Work out the finished part from the listing and answer in its coordinate system (mm). A direction names the side the tool comes from. Coordinates: 2 decimals unless noted, no trailing zeros. Order: outer loops, then holes, each group sorted by start corner. A loop starts at its lowest first (then second) coordinate and runs counter-clockwise, first axis right, second up. Notation, with made-up numbers: (66, -9) -> (101, -9) arc R26 ccw to (101, 5) -> close; hole circle Ø4 at (31.5, -3.75). An arc over 180 degrees is marked (long way). Use one line per item in the form item = value.
from build123d import *

# Parameters (mm, degrees)
BOSS_EXTRUDE1_DEPTH = 900
BOSS_EXTRUDE7_DEPTH = 154.432
BOSS_EXTRUDE9_DEPTH = 86.012287
FILLET1_R           = 2.54
FILLET2_R           = 2.54


with BuildPart() as part:
    # Sketch1 → Boss-Extrude1 (new body)
    with BuildSketch(Plane.XY):
        Polygon((0, -0.000240533), (154.432, -0.000240533), (154.432, -11.557240533), (81.28, -11.557240533), (81.28, -150.495240533), (154.432, -150.495240533), (154.432, -162.052240533), (0, -162.052240533), (0, -150.495240533), (73.152, -150.495240533), (73.152, -11.557240533), (0, -11.557240533), align=None)
    extrude(amount=BOSS_EXTRUDE1_DEPTH)

    # Sketch4 → Boss-Extrude7 (add)
    with BuildSketch(Plane(origin=(154.432, 0, 0), x_dir=(0, 0, -1), z_dir=(1, 0, 0))):
        Polygon((-900, -0.000240533), (-914.177712902, -162.052240533), (-900, -162.052240533), align=None)
    extrude(amount=-BOSS_EXTRUDE7_DEPTH)

    # Sketch6 → Boss-Extrude9 (add)
    with BuildSketch(Plane(origin=(0, 0, 0), x_dir=(-1, 0, 0), z_dir=(0, 0, -1))):
        Polygon((0, -11.557240533), (0, -0.000240533), (-154.432, -0.000240533), (-154.432, -11.557240533), (-81.28, -11.557240533), (-81.28, -150.495240533), (-154.432, -150.495240533), (-154.432, -162.052240533), (0, -162.052240533), (0, -150.495240533), (-73.152, -150.495240533), (-73.152, -11.557240533), align=None)
    extrude(amount=BOSS_EXTRUDE9_DEPTH)

    # Fillet1
    fillet1_edges = [part.edges().sort_by_distance(p)[0] for p in [
        (36.576, -150.495240533, 900),
        (117.856, -150.495240533, 900),
        (117.856, -11.557240533, 900),
        (77.216, -162.052240533, 914.177712902),
        (77.216, -0.000240533, 900),
        (36.576, -11.557240533, 900),
    ]]
    fillet(fillet1_edges, radius=FILLET1_R)

    # Fillet2
    fillet2_edges = [part.edges().sort_by_distance(p)[0] for p in [
        (77.216, -162.052240533, -86.012287),
    ]]
    fillet(fillet2_edges, radius=FILLET2_R)


solid = part.part
(1) Which of the six approach directions +Z, -Z, +X, -X, +Y, -Y give full straight-line access (tool end or side, diameter ignored) to faces 1 (the flat face through (81.28, -80, 414)), 2 (the flat face through (78, -56, -86.012)), 3 (the flat face through (37, -82, 900))?
Data:
face_1 = -Z, +X
face_2 = -Z, +X, -X, +Y, -Y
face_3 = -Z, -X
(2) Each of these flat-tipped pins is pushed along its axis until it touches: P1, Ø3, axis at y = -54, z = 795.5, coming from the +X side; P2, Ø2, axis at y = -144.5, z = 809, coming from the -X side. Where does it stop, or does it pass through?
Data:
P1 = 81.28
P2 = 73.15
(3) Section B-B on x = 143 is taken. Write down the section's boundary in (y, z).
Data:
outline = (-162.05, -83.47) arc R2.54 ccw to (-159.51, -86.01) -> (-150.5, -86.01) -> (-150.5, 897.46) arc R2.54 cw to (-147.96, 900) -> (-14.1, 900) arc R2.54 cw to (-11.56, 897.46) -> (-11.56, -86.01) -> (0, -86.01) -> (0, 897.67) arc R2.54 ccw to (-2.32, 900.2) -> (-159.29, 913.94) arc R2.54 ccw to (-162.05, 911.41) -> close
(4) Section D-D on y = -23.5 is taken. Write down the section's boundary in (x, z), plus the area to 3 significant figures.
Data:
outline = (0, 900) -> (73.15, 900) -> (73.15, -86.01) -> (81.28, -86.01) -> (81.28, 900) -> (154.43, 900) -> (154.43, 902.06) -> (0, 902.06) -> close
area = 8,330 mm²
(5) Section C-C on y = -80 is taken. Write down the section's boundary in (x, z), plus the area to 3 significant figures.
Data:
outline = (0, 900) -> (73.15, 900) -> (73.15, -86.01) -> (81.28, -86.01) -> (81.28, 900) -> (154.43, 900) -> (154.43, 907) -> (0, 907) -> close
area = 9,100 mm²
(6) The mould has two halves that part along Y. Classify faces 4 (the flat face through (37, -11.557, 413)), 5 (the flat face through (0, -153, 416)), 6 (the flat face through (78, -162.052, 421)): released by +Y, released by -Y, zero draft, split by the parting line, or undercut.
Data:
face_4 = undercut
face_5 = zero draft
face_6 = released by -Y
(7) Section A-A on z = 719.5 is taken. Write down the section's boundary in (x, y), plus the area to 3 significant figures.
Data:
outline = (0, -162.05) -> (154.43, -162.05) -> (154.43, -150.5) -> (81.28, -150.5) -> (81.28, -11.56) -> (154.43, -11.56) -> (154.43, 0) -> (0, 0) -> (0, -11.56) -> (73.15, -11.56) -> (73.15, -150.5) -> (0, -150.5) -> close
area = 4,700 mm²
(8) Straight lines are drawn through the part: line 1 along Y through (x, z) = (142, 309); line 2 along X through (y, z) = (-32.5, 761.5); line 3 along Z through (x, y) = (14.5, -23.5). For each, find the intervals that lie inside material, in ascending order.
Data:
line_1 = -162.05 to -150.5, -11.56 to 0
line_2 = 73.15 to 81.28
line_3 = 900 to 902.06
